```python
from build123d import *

# Parameters (mm, degrees)
BOSS_EXTRUDE1_DEPTH     = 13
SKETCH6_W               = 6
SKETCH6_H               = 5
BOSS_EXTRUDE4_DEPTH     = 5.6
SKETCH16_W              = 6
SKETCH16_H              = 8
BOSS_EXTRUDE5_DEPTH     = 0.1
CUT_EXTRUDE6_DEPTH      = 4
CUT_EXTRUDE6_DEPTH_BACK = 3.6
SKETCH15_R              = 1.3
CUT_EXTRUDE7_DEPTH      = 8.7202
CUT_EXTRUDE8_START      = -0.2202
SKETCH19_W              = 6
SKETCH19_H              = 8
SKETCH19_R              = 1.3
CUT_EXTRUDE8_DEPTH      = 0.2202
SKETCH12_R              = 1.2
CUT_EXTRUDE5_DEPTH      = 6
CHAMFER1_SIZE           = 0.2
SKETCH21_R              = 1.2
BOSS_EXTRUDE6_DEPTH     = 2.5
SKETCH24_W              = 6
SKETCH24_H              = 5.5
CUT_EXTRUDE10_DEPTH     = 8.5
SKETCH25_W              = 6
SKETCH25_H              = 7
BOSS_EXTRUDE8_DEPTH     = 12.9
SKETCH26_W              = 6
SKETCH26_H              = 7.39
BOSS_EXTRUDE9_DEPTH     = 3
SKETCH30_R              = 1.2
CUT_EXTRUDE13_DEPTH     = 8
SKETCH31_W              = 7
SKETCH31_H              = 9
BOSS_EXTRUDE11_DEPTH    = 1
SKETCH32_W              = 7
SKETCH32_H              = 9
BOSS_EXTRUDE12_DEPTH    = 1
BOSS_EXTRUDE13_DEPTH    = 1
BOSS_EXTRUDE14_DEPTH    = 1
SKETCH35_W              = 10
SKETCH35_H              = 4.2
CUT_EXTRUDE14_DEPTH     = 10
BOSS_EXTRUDE15_DEPTH    = 6
SKETCH38_R              = 1.3
CUT_EXTRUDE15_DEPTH     = 4
SKETCH39_R              = 1.2
CUT_EXTRUDE16_DEPTH     = 10
SKETCH40_W              = 14
SKETCH40_H              = 1.5
CUT_EXTRUDE17_DEPTH     = 10
SKETCH41_W              = 6.5
SKETCH41_H              = 3.19
CUT_EXTRUDE18_DEPTH     = 1.5
CROQUIS3_W              = 8.5
CROQUIS3_H              = 8.726674232
CORTAR_EXTRUIR3_DEPTH   = 1


with BuildPart() as part:
    # Sketch1 → Boss-Extrude1 (new body)
    with BuildSketch(Plane.XY):
        Polygon((3, 3.05), (3, -2.253801214), (2.388188946, -2.95), (-2.388188946, -2.95), (-3, -2.253801214), (-3, 3.05), align=None)
    extrude(amount=BOSS_EXTRUDE1_DEPTH)

    # Sketch6 → Boss-Extrude4 (add)
    with BuildSketch(Plane(origin=(0, 3.05, 0), x_dir=(1, 0, 0), z_dir=(0, 1, 0))):
        with Locations((0, -2.5)):
            Rectangle(SKETCH6_W, SKETCH6_H)
    extrude(amount=BOSS_EXTRUDE4_DEPTH)

    # Sketch16 → Boss-Extrude5 (add)
    with BuildSketch(Plane(origin=(0, 3.05, 0), x_dir=(1, 0, 0), z_dir=(0, 1, 0))):
        with Locations((0, -9)):
            Rectangle(SKETCH16_W, SKETCH16_H)
    extrude(amount=BOSS_EXTRUDE5_DEPTH)

    # Sketch18 → Cut-Extrude6 (cut, two sides: drawn at the far end of the back side and taken through both)
    with BuildSketch(Plane(origin=(0, 0, 0), x_dir=(0, 0, -1), z_dir=(1, 0, 0)).offset(-CUT_EXTRUDE6_DEPTH_BACK)):
        with BuildLine():
            Line((-8.8572, -0.0702), (-12.8572, -0.0702))
            Line((-12.8572, -0.0702), (-13, -0.0702))
            Line((-13, -0.0702), (-13, -0.7))
            Line((-13, -0.7), (-12.8572, -0.7))
            Line((-12.8572, -0.7), (-12.7144, -0.7))
            add(Edge.make_bspline(
                [(-12.7144, -0.7), (-12.5198, -0.7), (-12.43, -0.9509)],
                knots=[0.103448276, 0.103448276, 0.103448276, 0.137931034, 0.137931034, 0.137931034], degree=2))
            add(Edge.make_bspline(
                [(-12.43, -0.9509), (-12.3594, -1.2388), (-12.13, -1.45), (-11.8572, -1.45)],
                knots=[0.137931034, 0.137931034, 0.137931034, 0.137931034, 0.172413793, 0.172413793, 0.172413793, 0.172413793], degree=3))
            add(Edge.make_bspline(
                [(-11.8572, -1.45), (-11.5844, -1.45), (-11.355, -1.2388), (-11.2844, -0.9509)],
                knots=[0.172413793, 0.172413793, 0.172413793, 0.172413793, 0.206896552, 0.206896552, 0.206896552, 0.206896552], degree=3))
            add(Edge.make_bspline(
                [(-11.2844, -0.9509), (-11.1946, -0.7), (-11, -0.7)],
                knots=[0.206896552, 0.206896552, 0.206896552, 0.24137931, 0.24137931, 0.24137931], degree=2))
            Line((-11, -0.7), (-10.8572, -0.7))
            Line((-10.8572, -0.7), (-10.7144, -0.7))
            add(Edge.make_bspline(
                [(-10.7144, -0.7), (-10.5198, -0.7), (-10.43, -0.9509)],
                knots=[0.310344828, 0.310344828, 0.310344828, 0.344827586, 0.344827586, 0.344827586], degree=2))
            add(Edge.make_bspline(
                [(-10.43, -0.9509), (-10.3594, -1.2388), (-10.13, -1.45), (-9.8572, -1.45)],
                knots=[0.344827586, 0.344827586, 0.344827586, 0.344827586, 0.379310345, 0.379310345, 0.379310345, 0.379310345], degree=3))
            add(Edge.make_bspline(
                [(-9.8572, -1.45), (-9.5844, -1.45), (-9.355, -1.2388), (-9.2844, -0.9509)],
                knots=[0.379310345, 0.379310345, 0.379310345, 0.379310345, 0.413793103, 0.413793103, 0.413793103, 0.413793103], degree=3))
            add(Edge.make_bspline(
                [(-9.2844, -0.9509), (-9.1946, -0.7), (-9, -0.7)],
                knots=[0.413793103, 0.413793103, 0.413793103, 0.448275862, 0.448275862, 0.448275862], degree=2))
            Line((-9, -0.7), (-8.8572, -0.7))
            Line((-8.8572, -0.7), (-8.7144, -0.7))
            add(Edge.make_bspline(
                [(-8.7144, -0.7), (-8.5198, -0.7), (-8.43, -0.9509)],
                knots=[0.517241379, 0.517241379, 0.517241379, 0.551724138, 0.551724138, 0.551724138], degree=2))
            add(Edge.make_bspline(
                [(-8.43, -0.9509), (-8.3594, -1.2388), (-8.13, -1.45), (-7.8572, -1.45)],
                knots=[0.551724138, 0.551724138, 0.551724138, 0.551724138, 0.586206897, 0.586206897, 0.586206897, 0.586206897], degree=3))
            add(Edge.make_bspline(
                [(-7.8572, -1.45), (-7.5844, -1.45), (-7.355, -1.2388), (-7.2844, -0.9509)],
                knots=[0.586206897, 0.586206897, 0.586206897, 0.586206897, 0.620689655, 0.620689655, 0.620689655, 0.620689655], degree=3))
            add(Edge.make_bspline(
                [(-7.2844, -0.9509), (-7.1946, -0.7), (-7, -0.7)],
                knots=[0.620689655, 0.620689655, 0.620689655, 0.655172414, 0.655172414, 0.655172414], degree=2))
            Line((-7, -0.7), (-6.8572, -0.7))
            Line((-6.8572, -0.7), (-6.7144, -0.7))
            add(Edge.make_bspline(
                [(-6.7144, -0.7), (-6.5198, -0.7), (-6.43, -0.9509)],
                knots=[0.724137931, 0.724137931, 0.724137931, 0.75862069, 0.75862069, 0.75862069], degree=2))
            add(Edge.make_bspline(
                [(-6.43, -0.9509), (-6.3594, -1.2388), (-6.13, -1.45), (-5.8572, -1.45)],
                knots=[0.75862069, 0.75862069, 0.75862069, 0.75862069, 0.793103448, 0.793103448, 0.793103448, 0.793103448], degree=3))
            add(Edge.make_bspline(
                [(-5.8572, -1.45), (-5.5844, -1.45), (-5.355, -1.2388), (-5.2844, -0.9509)],
                knots=[0.793103448, 0.793103448, 0.793103448, 0.793103448, 0.827586207, 0.827586207, 0.827586207, 0.827586207], degree=3))
            add(Edge.make_bspline(
                [(-5.2844, -0.9509), (-5.1946, -0.7), (-5, -0.7)],
                knots=[0.827586207, 0.827586207, 0.827586207, 0.862068966, 0.862068966, 0.862068966], degree=2))
            Line((-5, -0.7), (-5, -0.0702))
            Line((-5, -0.0702), (-8.8572, -0.0702))
        make_face()
    extrude(amount=CUT_EXTRUDE6_DEPTH + CUT_EXTRUDE6_DEPTH_BACK, mode=Mode.SUBTRACT)

    # Sketch15 → Cut-Extrude7 (cut)
    with BuildSketch(Plane(origin=(0, 8.65, 0), x_dir=(1, 0, 0), z_dir=(0, 1, 0))):
        with Locations(Location((0, -10.8572, 0), (0, 0, 180))):
            Circle(SKETCH15_R)
        with Locations(Location((0, -6.8572, 0), (0, 0, 180))):
            Circle(SKETCH15_R)
    extrude(amount=-CUT_EXTRUDE7_DEPTH, mode=Mode.SUBTRACT)

    # Sketch19 → Cut-Extrude8 (cut)
    with BuildSketch(Plane.XZ.offset(0.0702).offset(CUT_EXTRUDE8_START)):
        with Locations((0, 9)):
            Rectangle(SKETCH19_W, SKETCH19_H)
        with Locations(Location((0, 10.8572, 0), (0, 0, 180))):
            Circle(SKETCH19_R, mode=Mode.SUBTRACT)
        with Locations(Location((0, 6.8572, 0), (0, 0, 180))):
            Circle(SKETCH19_R, mode=Mode.SUBTRACT)
    extrude(amount=CUT_EXTRUDE8_DEPTH, mode=Mode.SUBTRACT)

    # Sketch12 → Cut-Extrude5 (cut)
    with BuildSketch(Plane.XY.offset(5)):
        with Locations((0, 5.85)):
            Circle(SKETCH12_R)
    extrude(amount=-CUT_EXTRUDE5_DEPTH, mode=Mode.SUBTRACT)

    # Chamfer1
    chamfer1_edges = [part.edges().sort_by_distance(p)[0] for p in [
        (-2.694094473, -2.601900607, 13),
        (0, -2.95, 13),
        (2.694094473, -2.601900607, 13),
        (3, 1.65, 13),
        (3, -1.476900607, 13),
        (-3, -1.476900607, 13),
        (-3, 1.65, 13),
    ]]
    chamfer(chamfer1_edges, length=CHAMFER1_SIZE)

    # Sketch21 → Boss-Extrude6 (add)
    with BuildSketch(Plane(origin=(0, 0, 0), x_dir=(-1, 0, 0), z_dir=(0, 0, -1))):
        Polygon((-2.388188946, -2.95), (2.388188946, -2.95), (3, -2.253801214), (3, 8.65), (-3, 8.65), (-3, -2.253801214), align=None)
        with Locations(Location((0, 5.85, 0), (0, 0, 180))):
            Circle(SKETCH21_R, mode=Mode.SUBTRACT)
    extrude(amount=BOSS_EXTRUDE6_DEPTH)

    # Sketch24 → Cut-Extrude10 (cut)
    with BuildSketch(Plane.XY.offset(5)):
        with Locations((0, 5.9)):
            Rectangle(SKETCH24_W, SKETCH24_H)
    extrude(amount=-CUT_EXTRUDE10_DEPTH, mode=Mode.SUBTRACT)

    # Sketch25 → Boss-Extrude8 (add)
    with BuildSketch(Plane(origin=(0, 3.15, 0), x_dir=(1, 0, 0), z_dir=(0, 1, 0))):
        with Locations((0, -1)):
            Rectangle(SKETCH25_W, SKETCH25_H)
    extrude(amount=BOSS_EXTRUDE8_DEPTH)

    # Sketch26 → Boss-Extrude9 (add)
    with BuildSketch(Plane(origin=(0, 0, -2.5), x_dir=(-1, 0, 0), z_dir=(0, 0, -1))):
        with Locations((0, 12.355)):
            Rectangle(SKETCH26_W, SKETCH26_H)
    extrude(amount=BOSS_EXTRUDE9_DEPTH)

    # Sketch30 → Cut-Extrude13 (cut)
    with BuildSketch(Plane(origin=(0, 0, -2.5), x_dir=(-1, 0, 0), z_dir=(0, 0, -1))):
        with Locations((0, 5.9)):
            Circle(SKETCH30_R)
    extrude(amount=-CUT_EXTRUDE13_DEPTH, mode=Mode.SUBTRACT)

    # Sketch31 → Boss-Extrude11 (add)
    with BuildSketch(Plane(origin=(3, 0, 0), x_dir=(0, 0, -1), z_dir=(1, 0, 0))):
        with Locations((-1, 7.65)):
            Rectangle(SKETCH31_W, SKETCH31_H)
    extrude(amount=BOSS_EXTRUDE11_DEPTH)

    # Sketch32 → Boss-Extrude12 (add)
    with BuildSketch(Plane.ZY.offset(3)):
        with Locations((1, 7.65)):
            Rectangle(SKETCH32_W, SKETCH32_H)
    extrude(amount=BOSS_EXTRUDE12_DEPTH)

    # Sketch33 → Boss-Extrude13 (add)
    with BuildSketch(Plane(origin=(3, 0, 0), x_dir=(0, 0, -1), z_dir=(1, 0, 0))):
        Polygon((2.5, 12.15), (2.5, 8.66), (5.5, 8.66), (5.5, 16.05), (-4.5, 16.05), (-4.5, 12.15), align=None)
    extrude(amount=BOSS_EXTRUDE13_DEPTH)

    # Sketch34 → Boss-Extrude14 (add)
    with BuildSketch(Plane.ZY.offset(3)):
        Polygon((-2.5, 12.15), (4.5, 12.15), (4.5, 16.05), (-5.5, 16.05), (-5.5, 8.66), (-2.5, 8.66), align=None)
    extrude(amount=BOSS_EXTRUDE14_DEPTH)

    # Sketch35 → Cut-Extrude14 (cut)
    with BuildSketch(Plane.ZY.offset(4)):
        with Locations((-0.5, 13.95)):
            Rectangle(SKETCH35_W, SKETCH35_H)
    extrude(amount=-CUT_EXTRUDE14_DEPTH, mode=Mode.SUBTRACT)

    # Sketch36 → Boss-Extrude15 (add)
    with BuildSketch(Plane.ZY.offset(4)):
        Polygon((4.5, 3.15), (4.5, 11.85), (-5.5, 11.85), (-5.5, 8.66), (-2.5, 8.66), (-2.5, 3.15), align=None)
    extrude(amount=BOSS_EXTRUDE15_DEPTH)

    # Sketch38 → Cut-Extrude15 (cut)
    with BuildSketch(Plane(origin=(0, 11.85, 0), x_dir=(1, 0, 0), z_dir=(0, 1, 0))):
        with Locations(Location((0.5, -1, 0), (0, 0, 270))):
            Circle(SKETCH38_R)
    extrude(amount=-CUT_EXTRUDE15_DEPTH, mode=Mode.SUBTRACT)

    # Sketch39 → Cut-Extrude16 (cut)
    with BuildSketch(Plane(origin=(0, 11.85, 0), x_dir=(1, 0, 0), z_dir=(0, 1, 0))):
        with Locations(Location((-6.5, -1, 0), (0, 0, 270))):
            Circle(SKETCH39_R)
    extrude(amount=-CUT_EXTRUDE16_DEPTH, mode=Mode.SUBTRACT)

    # Sketch40 → Cut-Extrude17 (cut)
    with BuildSketch(Plane(origin=(0, 11.85, 0), x_dir=(1, 0, 0), z_dir=(0, 1, 0))):
        with Locations((-3, 4.75)):
            Rectangle(SKETCH40_W, SKETCH40_H)
    extrude(amount=-CUT_EXTRUDE17_DEPTH, mode=Mode.SUBTRACT)

    # Sketch41 → Cut-Extrude18 (cut)
    with BuildSketch(Plane(origin=(0, 0, -4), x_dir=(-1, 0, 0), z_dir=(0, 0, -1))):
        with Locations((6.75, 10.255)):
            Rectangle(SKETCH41_W, SKETCH41_H)
    extrude(amount=-CUT_EXTRUDE18_DEPTH, mode=Mode.SUBTRACT)

    # Croquis3 → Cortar-Extruir3 (cut)
    with BuildSketch(Plane(origin=(4, 0, 0), x_dir=(0, 0, -1), z_dir=(1, 0, 0))):
        with Locations((-0.25, 7.486662884)):
            Rectangle(CROQUIS3_W, CROQUIS3_H)
    extrude(amount=-CORTAR_EXTRUIR3_DEPTH, mode=Mode.SUBTRACT)


solid = part.part
```
Read the model definition and answer for the solid it produces. Units are mm, in the model's axes. A direction names the side the tool comes from. Coordinates: 2 decimals unless noted, no trailing zeros. Order: outer loops, then holes, each group sorted by start corner. A loop starts at its lowest first (then second) coordinate and runs counter-clockwise, first axis right, second up. Notation, with made-up numbers: (85.5, -38.75) - (140.5, -38.75) arc R30 ccw to (140.5, -5.75) - close; hole circle Ø4 at (-18.5, 22.5). An arc over 180 degrees is marked (long way). Answer as a JSON object with one key per item and string values. Group by question number.
Item 1: Consider probe 1 along Z at (x, y) = (0, 1); probe 2 along Y at (x, z) = (0, 1.5); probe 3 along X at (y, z) = (-1, 3.25). Determine where each line is inside the solid, lowest interval first. Write a range as from..to.
Item 2: Section B-B (y = 5.9) is taken. Give the vertices of the cut face in (x, z), plus the area to 3 significant figures.
Item 3: Section C-C (x = -6.5) is taken. Give the vertices of the cut face in (y, z).
Item 4: Section A-A (z = 1) is taken. Give the vertices of the cut face in (x, y), plus the area to 3 significant figures.
Item 5: Flat-ended cylindrical pins translate along their axes: P1, Ø2.5, axis at x = 0, z = 10.86, coming from the +Y side; P2, Ø0.8, axis at x = 0, z = -3, coming from the -Y side; P3, Ø4, axis at y = 1, z = 5, coming from the -X side. Find the tip coordinate at first contact, or state that the pin passes through.
Item 6: A tool of negligible diameter and unlimited length cuts with its end or side. For faces 4 (the face through (-0.29, 9.88, -0.03)), 5 (the face through (0, 3.15, 9)), 6 (the face through (0, 8.66, -3)), 7 (the face through (0, 0.15, 9)), from which of +Z, -Z, +X, -X, +Y, -Y can it reach the whole face along a straight path? Write none if from no direction.
Item 7: Section D-D (z = -1.25) is taken. Give the vertices of the cut face in (x, y), plus the area to 3 significant figures.
Item 8: The mould has two halves that part along Y. Classify faces 1 (the face through (-10, 8, 1)), 2 (the face through (0.26, 4.73, 0.95)), 3 (the face through (1, 7.85, 1)): +Y half, -Y half, draft (parallel to the pull), parting line (faces both ways), or undercut.
Results are:
{
 "1": {"probe 1": "z = -2.5..5.56, 8.16..9.56, 12.16..13", "probe 2": "y = -2.95..4.7, 7.1..7.85", "probe 3": "x = -3..3"},
 "2": {"outline": "(-10, -2.5) - (-1.2, -2.5) - (-1.2, 4.5) - (-10, 4.5) - close; (1.2, -2.5) - (3, -2.5) - (3, 4.5) - (1.2, 4.5) - close; hole circle Ø2.4 at (-6.5, 1)", "area": "69.7 mm^2"},
 "3": {"outline": "(3.15, -2.5) - (11.85, -2.5) - (11.85, -0.2) - (3.15, -0.2) - close; (3.15, 2.2) - (11.85, 2.2) - (11.85, 4.5) - (3.15, 4.5) - close"},
 "4": {"outline": "(-10, 3.15) - (-7.7, 3.15) - (-7.7, 11.85) - (-10, 11.85) - close; (-5.3, 3.15) - (-3, 3.15) - (-3, -2.25) - (-2.39, -2.95) - (2.39, -2.95) - (3, -2.25) - (3, 11.85) - (1.8, 11.85) - (1.8, 7.85) - (-0.8, 7.85) - (-0.8, 11.85) - (-5.3, 11.85) - close; hole circle Ø2.4 at (0, 5.9)", "area": "113 mm^2"},
 "5": {"P1": "stops at y = -0.7", "P2": "stops at y = 8.66", "P3": "stops at x = -3"},
 "6": {"face 4": "+Y", "face 5": "+Z, +X, -X, +Y", "face 6": "-Z, +X, -X, -Y", "face 7": "+Z, +X, -X"},
 "7": {"outline": "(-10, 3.15) - (-3, 3.15) - (-3, -2.25) - (-2.39, -2.95) - (2.39, -2.95) - (3, -2.25) - (3, 11.85) - (-10, 11.85) - close; hole circle Ø2.4 at (0, 5.9)", "area": "145 mm^2"},
 "8": {"face 1": "draft", "face 2": "undercut", "face 3": "+Y half"}
}
